Input: part model. Units: mm. Frame: model coordinates. Coordinates: 2 decimals unless noted, no trailing zeros. Write each loop counter-clockwise with the first axis right and the second up, starting at its lowest first coordinate (ties: lowest second). Pieces come first, ordered by that corner, then holes. Notation, with made-up numbers: M 19.5,-29 L 45.5,-29 A8 cw 45.5,-15 Z; hole C 68,68 d3. An arc over 180 degrees is marked long. Answer as a JSON object with one key per item and string values. Group by question number.
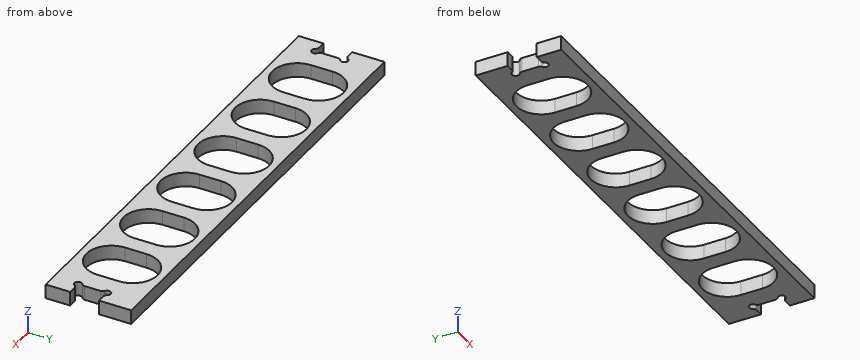
from build123d import *

# Parameters (mm, degrees)
F0_W     = 406.4
F0_H     = 76.2
F1_DEPTH = 12.7
F3_DEPTH = 25.4
F5_DEPTH = 25.4


with BuildPart() as f1:
    # F0 (on Top) → F1 (new body)
    with BuildSketch(Plane.XY):
        with Locations((203.2, 38.1)):
            Rectangle(F0_W, F0_H)
    extrude(amount=F1_DEPTH)

    # F2 (on face) → F3 (cut)
    with BuildSketch(Plane.XY.offset(12.7)):
        with BuildLine():
            Line((7.054568, 47.625), (0, 47.625))
            Line((0, 47.625), (0, 21.844))
            Line((0, 21.844), (7.054568, 21.844))
            ThreePointArc((7.054568, 21.844), (8.657556, 21.40963), (9.821937, 20.225373))
            ThreePointArc((9.821937, 20.225373), (15.034867, 19.509133), (14.318627, 24.722063))
            ThreePointArc((14.318627, 24.722063), (13.13437, 25.886444), (12.7, 27.489432))
            Line((12.7, 27.489432), (12.7, 41.979568))
            ThreePointArc((12.7, 41.979568), (13.13437, 43.582556), (14.318627, 44.746937))
            ThreePointArc((14.318627, 44.746937), (15.034867, 49.959867), (9.821937, 49.243627))
            ThreePointArc((9.821937, 49.243627), (8.657556, 48.05937), (7.054568, 47.625))
        make_face()
        with BuildLine():
            Line((393.7, 41.979568), (393.7, 27.489432))
            ThreePointArc((393.7, 27.489432), (393.26563, 25.886444), (392.081373, 24.722063))
            ThreePointArc((392.081373, 24.722063), (391.365133, 19.509133), (396.578063, 20.225373))
            ThreePointArc((396.578063, 20.225373), (397.742444, 21.40963), (399.345432, 21.844))
            Line((399.345432, 21.844), (406.4, 21.844))
            Line((406.4, 21.844), (406.4, 47.625))
            Line((406.4, 47.625), (399.345432, 47.625))
            ThreePointArc((399.345432, 47.625), (397.742444, 48.05937), (396.578063, 49.243627))
            ThreePointArc((396.578063, 49.243627), (391.365133, 49.959867), (392.081373, 44.746937))
            ThreePointArc((392.081373, 44.746937), (393.26563, 43.582556), (393.7, 41.979568))
        make_face()
    extrude(amount=-F3_DEPTH, mode=Mode.SUBTRACT)

    # F4 (on face) → F5 (cut)
    with BuildSketch(Plane.XY.offset(12.7)):
        with BuildLine():
            ThreePointArc((31.75, 28.575), (53.975, 6.35), (76.2, 28.575))
            Line((76.2, 28.575), (76.2, 47.625))
            ThreePointArc((76.2, 47.625), (53.975, 69.85), (31.75, 47.625))
            Line((31.75, 47.625), (31.75, 28.575))
        make_face()
        with BuildLine():
            Line((91.44, 47.625), (91.44, 28.575))
            ThreePointArc((91.44, 28.575), (113.665, 6.35), (135.89, 28.575))
            Line((135.89, 28.575), (135.89, 47.625))
            ThreePointArc((135.89, 47.625), (113.665, 69.85), (91.44, 47.625))
        make_face()
        with BuildLine():
            Line((151.13, 47.625), (151.13, 28.575))
            ThreePointArc((151.13, 28.575), (173.355, 6.35), (195.58, 28.575))
            Line((195.58, 28.575), (195.58, 47.625))
            ThreePointArc((195.58, 47.625), (173.355, 69.85), (151.13, 47.625))
        make_face()
        with BuildLine():
            Line((210.82, 47.625), (210.82, 28.575))
            ThreePointArc((210.82, 28.575), (233.045, 6.35), (255.27, 28.575))
            Line((255.27, 28.575), (255.27, 47.625))
            ThreePointArc((255.27, 47.625), (233.045, 69.85), (210.82, 47.625))
        make_face()
        with BuildLine():
            Line((270.51, 47.625), (270.51, 28.575))
            ThreePointArc((270.51, 28.575), (292.735, 6.35), (314.96, 28.575))
            Line((314.96, 28.575), (314.96, 47.625))
            ThreePointArc((314.96, 47.625), (292.735, 69.85), (270.51, 47.625))
        make_face()
        with BuildLine():
            Line((330.2, 47.625), (330.2, 28.575))
            ThreePointArc((330.2, 28.575), (352.425, 6.35), (374.65, 28.575))
            Line((374.65, 28.575), (374.65, 47.625))
            ThreePointArc((374.65, 47.625), (352.425, 69.85), (330.2, 47.625))
        make_face()
    extrude(amount=-F5_DEPTH, mode=Mode.SUBTRACT)


solid = f1.part
Q1. Section C-C, the plane z = 3. State how many separate pieces and enclosed holes the cut face has, and give its area (3 significant figures).
Q2. Section B-B, the plane x = 305.5. Return the cut outline in (y, z).
Q3. Line query: line 1 (Y direction, x = 171.5, z = 2); line 2 (Y direction, x = 185, z = 7) (3 decimals). Output: solid intervals per line, ascending. Write a range as from..to.
Q4. Pin query (flat end, axial travel): pin 1 Ø10.5 at (x, y) = (393.7, 47.625) entering from +Z; pin 2 Ø1.5 at (x, y) = (272, 34.5) entering from +Z (3 decimals); pin 3 Ø6.5 at (y, z) = (34.5, 8.5) entering from -X; pin 4 Ø6.5 at (y, z) = (34.5, 9) entering from +X. Return the tip coordinate at first contact, or that it passes through.
Q5. Section D-D, the plane x = 102.5. Return the cut outline in (y, z), and give its area (3 significant figures).
Q6. Section A-A, the plane y = 34. Return the cut outline in (x, z).
Filled in:
{
 "1": {"separate pieces": "1", "enclosed holes": "6", "area": "15,800 mm^2"},
 "2": {"outline": "M 0,0 L 10.38,0 L 10.38,12.7 L 0,12.7 Z; M 65.82,0 L 76.2,0 L 76.2,12.7 L 65.82,12.7 Z"},
 "3": {"line 1": "0..6.43, 69.77..76.2", "line 2": "0..9.645, 66.555..76.2"},
 "4": {"pin 1": "z = 12.7", "pin 2": "through", "pin 3": "x = 12.7", "pin 4": "x = 393.7"},
 "5": {"outline": "M 0,0 L 9.36,0 L 9.36,12.7 L 0,12.7 Z; M 66.84,0 L 76.2,0 L 76.2,12.7 L 66.84,12.7 Z", "area": "238 mm^2"},
 "6": {"outline": "M 12.7,0 L 31.75,0 L 31.75,12.7 L 12.7,12.7 Z; M 76.2,0 L 91.44,0 L 91.44,12.7 L 76.2,12.7 Z; M 135.89,0 L 151.13,0 L 151.13,12.7 L 135.89,12.7 Z; M 195.58,0 L 210.82,0 L 210.82,12.7 L 195.58,12.7 Z; M 255.27,0 L 270.51,0 L 270.51,12.7 L 255.27,12.7 Z; M 314.96,0 L 330.2,0 L 330.2,12.7 L 314.96,12.7 Z; M 374.65,0 L 393.7,0 L 393.7,12.7 L 374.65,12.7 Z"}
}
